The model under review builds one solid part; all positions refer to its coordinate system, in mm. Give positions to 0.01 mm unless a question says otherwise; leave off trailing zeros. Order: outer loops, then holes, each group sorted by start corner. A loop starts at its lowest first (then second) coordinate and runs counter-clockwise, first axis right, second up. Notation, with made-up numbers: (73, -39) - (86, -39) arc R7 cw to (86, -30) - close; hole circle Ø11 at (-17, -28). An arc over 180 degrees is marked (long way). Write item = value, one per line. Start each with the question number.
1. We need section C-C, the plane z = 1.8. State how many separate pieces and enclosed holes the cut face has, and give its area (3 significant figures).
2. For P1, Ø1, axis at x = 36, z = 1.5, coming from the -Y side; P2, Ø0.8, axis at y = 4.5, z = 1, coming from the -X side; P3, Ø1.5, axis at x = 33.5, z = 1.5, coming from the +Y side, all flat-tipped, find the tip position at first contact; note any pin that passes through.
3. We need section A-A, the plane y = -7. Give the boundary of the cut face in (x, z), and give its area (3 significant figures).
4. We need section B-B, the plane y = 0.5. Give the boundary of the cut face in (x, z).
5. Wall thickness on probe 1 along Y at (x, z) = (53.5, 0.8); probe 2 along X at (y, z) = (-8, 2.5); probe 3 along X at (y, z) = (2, 1): over which ranges is each line inside the solid? List them lowest first.
6. We need section D-D, the plane x = 14. Give the boundary of the cut face in (y, z), and give its area (3 significant figures).
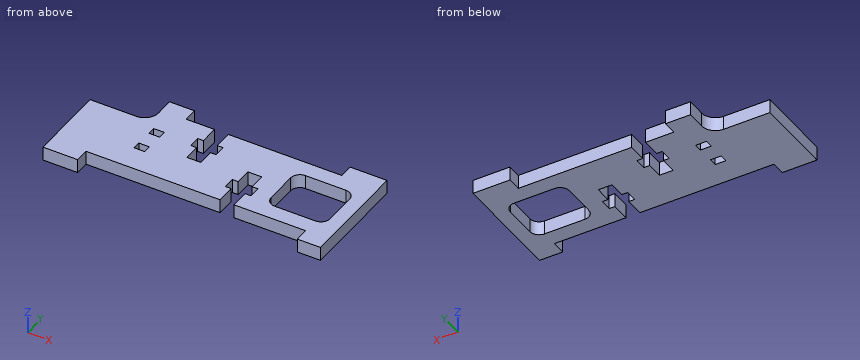
from build123d import *

# Parameters (mm, degrees)
SKETCH_1_W      = 2.3276
SKETCH_1_H      = 1.694
EXTRUDE_1_DEPTH = 3


with BuildPart() as part:
    # 草图1 → 凸台-拉伸1 (new body)
    with BuildSketch(Plane.XY.offset(3)):
        with BuildLine():
            Line((23.2531, 5.583631793), (24.503, 5.583631793))
            Line((24.503, 5.583631793), (24.503, 9.583631793))
            Line((24.503, 9.583631793), (18.3721, 9.583631793))
            Line((18.3721, 9.583631793), (18.3721, 12.583631793))
            Line((18.3721, 12.583631793), (12.9991, 12.583631793))
            Line((12.9991, 12.583631793), (12.9991, 8.582631793))
            ThreePointArc((12.9991, 8.582631793), (12.120420344, 6.461311449), (9.9991, 5.582631793))
            Line((9.9991, 5.582631793), (0, 5.582631793))
            Line((0, 5.582631793), (0, -11.416368207))
            Line((0, -11.416368207), (7.4994, -11.416368207))
            Line((7.4994, -11.416368207), (7.4994, -8.416368207))
            Line((7.4994, -8.416368207), (36.5002, -8.416368207))
            Line((36.5002, -8.416368207), (36.5002, -4.416368207))
            Line((36.5002, -4.416368207), (35.2489, -4.416368207))
            Line((35.2489, -4.416368207), (35.2489, -1.916368207))
            Line((35.2489, -1.916368207), (36.5002, -1.916368207))
            Line((36.5002, -1.916368207), (36.5002, 1.583631793))
            Line((36.5002, 1.583631793), (39.5003, 1.583631793))
            Line((39.5003, 1.583631793), (39.5003, -1.916368207))
            Line((39.5003, -1.916368207), (40.7501, -1.916368207))
            Line((40.7501, -1.916368207), (40.7501, -4.416368207))
            Line((40.7501, -4.416368207), (39.5003, -4.416368207))
            Line((39.5003, -4.416368207), (39.5003, -8.416368207))
            Line((39.5003, -8.416368207), (54.9988, -8.416368207))
            Line((54.9988, -8.416368207), (54.9988, -11.416368207))
            Line((54.9988, -11.416368207), (59.9998, -11.416368207))
            Line((59.9998, -11.416368207), (59.9998, 12.583631793))
            Line((59.9998, 12.583631793), (51.9988, 12.583631793))
            Line((51.9988, 12.583631793), (51.9988, 9.583631793))
            Line((51.9988, 9.583631793), (27.5031, 9.583631793))
            Line((27.5031, 9.583631793), (27.5031, 5.583631793))
            Line((27.5031, 5.583631793), (28.7543, 5.583631793))
            Line((28.7543, 5.583631793), (28.7543, 3.083631793))
            Line((28.7543, 3.083631793), (27.5031, 3.083631793))
            Line((27.5031, 3.083631793), (27.5031, -0.416368207))
            Line((27.5031, -0.416368207), (24.503, -0.416368207))
            Line((24.503, -0.416368207), (24.503, 3.083631793))
            Line((24.503, 3.083631793), (23.2531, 3.083631793))
            Line((23.2531, 3.083631793), (23.2531, 5.583631793))
        make_face()
        with BuildLine():
            Line((46.2504, 6.082631793), (54.9998, 6.082631793))
            ThreePointArc((54.9998, 6.082631793), (56.414013562, 5.496845355), (56.9998, 4.082631793))
            Line((56.9998, 4.082631793), (56.9998, -2.916368207))
            ThreePointArc((56.9998, -2.916368207), (56.414013562, -4.330581769), (54.9998, -4.916368207))
            Line((54.9998, -4.916368207), (46.2504, -4.916368207))
            ThreePointArc((46.2504, -4.916368207), (44.836186438, -4.330581769), (44.2504, -2.916368207))
            Line((44.2504, -2.916368207), (44.2504, 4.082631793))
            ThreePointArc((44.2504, 4.082631793), (44.836186438, 5.496845355), (46.2504, 6.082631793))
        make_face(mode=Mode.SUBTRACT)
        with Locations((15.811, 3.177631793)):
            Rectangle(SKETCH_1_W, SKETCH_1_H, mode=Mode.SUBTRACT)
        with Locations((15.7586, -2.060368207)):
            Rectangle(SKETCH_1_W, SKETCH_1_H, mode=Mode.SUBTRACT)
    extrude(amount=-EXTRUDE_1_DEPTH)


solid = part.part
Model answer:
q1.separate_pieces = 1
q1.enclosed_holes = 3
q1.area = 890 mm2
q2.P1 = -8.42
q2.P2 = 0
q2.P3 = 9.58
q3.outline = (0, 0) - (36.5, 0) - (36.5, 3) - (0, 3) - close; (39.5, 0) - (60, 0) - (60, 3) - (39.5, 3) - close
q3.area = 171 mm2
q4.outline = (0, 0) - (24.5, 0) - (24.5, 3) - (0, 3) - close; (27.5, 0) - (36.5, 0) - (36.5, 3) - (27.5, 3) - close; (39.5, 0) - (44.25, 0) - (44.25, 3) - (39.5, 3) - close; (57, 0) - (60, 0) - (60, 3) - (57, 3) - close
q5.probe_1 = -8.42 to -4.92, 6.08 to 12.58
q5.probe_2 = 0 to 36.5, 39.5 to 60
q5.probe_3 = 0 to 24.5, 27.5 to 44.25, 57 to 60
q6.outline = (-8.42, 0) - (12.58, 0) - (12.58, 3) - (-8.42, 3) - close
q6.area = 63.0 mm2
